```python
from build123d import *

# Parameters (mm, degrees)
SKETCH1_R           = 2
BOSS_EXTRUDE1_DEPTH = 4
SKETCH2_W           = 2
SKETCH2_H           = 1
CUT_EXTRUDE1_DEPTH  = 4
CUT_EXTRUDE2_START  = -4
CUT_EXTRUDE2_DEPTH  = 4
CUT_EXTRUDE3_START  = -3
CUT_EXTRUDE3_DEPTH  = 3
CUT_EXTRUDE4_START  = -2
CUT_EXTRUDE4_DEPTH  = 2
CUT_EXTRUDE5_START  = -1
CUT_EXTRUDE5_DEPTH  = 1


# Read off the part's stored shape, not the designer's step: Cut-Extrude4
with BuildPart() as part:
    # Sketch1 → Boss-Extrude1 (new body)
    with BuildSketch(Plane.XY):
        with BuildLine():
            Line((4, -5), (-4, -5))
            Line((-4, -5), (-4, 0))
            ThreePointArc((-4, 0), (0, 4), (4, 0))
            Line((4, 0), (4, -5))
        make_face()
        Circle(SKETCH1_R, mode=Mode.SUBTRACT)
    extrude(amount=BOSS_EXTRUDE1_DEPTH)

    # Sketch2 → Cut-Extrude1 (cut)
    with BuildSketch(Plane.XY.offset(4)):
        with Locations((1, -4.5)):
            Rectangle(SKETCH2_W, SKETCH2_H)
    extrude(amount=-CUT_EXTRUDE1_DEPTH, mode=Mode.SUBTRACT)

    # Sketch3 → Cut-Extrude2 (cut)
    with BuildSketch(Plane.XY.offset(4).offset(CUT_EXTRUDE2_START)):
        with BuildLine():
            Line((1, 3.327826432), (-1, 3.327826432))
            Line((-1, 3.327826432), (-1, 3.872983346))
            ThreePointArc((-1, 3.872983346), (0, 4), (1, 3.872983346))
            Line((1, 3.872983346), (1, 3.327826432))
        make_face()
    extrude(amount=CUT_EXTRUDE2_DEPTH, mode=Mode.SUBTRACT)

    # Sketch5 → Cut-Extrude3 (cut)
    with BuildSketch(Plane.XY.offset(4).offset(CUT_EXTRUDE3_START)):
        with BuildLine():
            Line((4, 0), (-4, 0))
            ThreePointArc((-4, 0), (0, 4), (4, 0))
        make_face()
    extrude(amount=CUT_EXTRUDE3_DEPTH, mode=Mode.SUBTRACT)

    # Cut-Extrude4 outline → Cut-Extrude4 (cut)
    with BuildSketch(Plane.XY.offset(4).offset(CUT_EXTRUDE4_START)):
        with BuildLine():
            ThreePointArc((-3, -5), (-2.142135206, -2.878264494), (-0.028848782, -1.999791926))
            ThreePointArc((-0.028848782, -1.999791926), (-1.424376629, -1.403976929), (-2, 0))
            Line((-2, 0), (-4, 0))
            Line((-4, 0), (-4, -5))
            Line((-4, -5), (-3, -5))
        make_face()
    extrude(amount=CUT_EXTRUDE4_DEPTH, mode=Mode.SUBTRACT)

    # Sketch7 → Cut-Extrude5 (cut)
    with BuildSketch(Plane.XY.offset(4).offset(CUT_EXTRUDE5_START)):
        with BuildLine():
            Line((3, -1), (4, -1))
            Line((4, -1), (4, 0))
            Line((4, 0), (2, 0))
            ThreePointArc((2, 0), (1.403976929, -1.424376629), (-0.028848782, -1.999791926))
            ThreePointArc((-0.028848782, -1.999791926), (-1.173685148, -2.226867466), (-2.142135206, -2.878264494))
            Line((-2.142135206, -2.878264494), (0.857864794, -2.878264494))
            ThreePointArc((0.857864794, -2.878264494), (2.166117347, -2.209638468), (3, -1))
        make_face()
    extrude(amount=CUT_EXTRUDE5_DEPTH, mode=Mode.SUBTRACT)


solid = part.part
```
Work out the finished part from the listing and answer in its coordinate system (mm). A direction names the side the tool comes from. Coordinates: 2 decimals unless noted, no trailing zeros. Loops run counter-clockwise (first coordinate to the right, second up) from the corner with the lowest first, then second, coordinate; pieces in that order, holes last. Notation, with made-up numbers: M 10,72.25 L 16,72.25 A34 ccw 16,107.25 Z; hole C 65,34.25 d3. An arc over 180 degrees is marked long. Use CSV: the item, a comma, the result in double quotes. Start each with the question number.
(1) For faces 1 (the face through (0.1, -2.5, 0)), 2 (the face through (2.15, -2.223, 3.493)), 3 (the face through (0, 3.328, 0.5)), 4 (the face through (3.5, -1, 3.5)), 5 (the face through (2, -4.5, 2)), determine the directions among +Z, -Z, +X, -X, +Y, -Y from which every point of the face is accessible in a straight line to the end or side of a thin tool.
(2) Consider line 1 (Z direction, x = 0.5, y = 3.25); line 2 (Z direction, x = -0.5, y = -2.75); line 3 (Y direction, x = 3.5, z = 2.15). Determine where each line is inside the solid, lowest interval first.
(3) For a pull along X with two mould halves and no side action, classify faces 6 (the face through (3.14, 2.48, 0.49)), 7 (the face through (1, -4, 2)), 8 (the face through (-3, -2, 2)) as +X half, -X half, draft (parallel to the pull), parting line (faces both ways), or undercut.
(4) Find section B-B, the plane x = -0.5. Give the vertices of the cut face in (y, z).
(5) Find section C-C, the plane y = -0.25. Give the vertices of the cut face in (x, z), then the cut area to 3 significant figures.
(6) Find section A-A, the plane z = 0.85. Give the vertices of the cut face in (x, y), then the cut area to 3 significant figures.
(7) Find section D-D, the plane z = 2.4. Give the vertices of the cut face in (x, y).
(8) Given pin 1 Ø0.8 at (x, z) = (-0.5, 3.5) entering from +Y; pin 2 Ø0.5 at (x, z) = (-3, 1.5) entering from +Y; pin 3 Ø1.1 at (y, z) = (-4.5, 3) entering from -X, each flat-ended and moving along its own axis, determine where each tip first touches the part or whether it passes through.
Recorded:
1,face 1,"-Z, +X, -X, +Y, -Y"
1,face 2,"+Z, -X, +Y"
1,face 3,"+Z, -Z, +Y"
1,face 4,"+Z, +X, -X, +Y"
1,face 5,"+Z, -Z, -Y"
2,line 1,"z = 0 to 1"
2,line 2,"z = 0 to 3"
2,line 3,"y = -5 to 0"
3,face 6,"+X half"
3,face 7,"undercut"
3,face 8,"draft"
4,outline,"M -5,0 L -1.94,0 L -1.94,2 L -2.04,2 L -2.04,3 L -2.88,3 L -2.88,4 L -5,4 Z; M 1.94,0 L 3.33,0 L 3.33,1 L 1.94,1 Z"
5,outline,"M -4,0 L -1.98,0 L -1.98,2 L -4,2 Z; M 1.98,0 L 4,0 L 4,3 L 1.98,3 Z"
5,area,"10.1 mm^2"
6,outline,"M -4,-5 L 0,-5 L 0,-4 L 2,-4 L 2,-5 L 4,-5 L 4,0 A4 ccw 1,3.87 L 1,3.33 L -1,3.33 L -1,3.87 A4 ccw -4,0 Z; hole C 0,0 d4"
6,area,"49.3 mm^2"
7,outline,"M -3,-5 L 0,-5 L 0,-4 L 2,-4 L 2,-5 L 4,-5 L 4,0 L 2,0 A2 cw -0.03,-2 A2.96 ccw Z"
8,pin 1,"stops at y = -2.88"
8,pin 2,"stops at y = 0"
8,pin 3,"stops at x = -3"
